from build123d import *

# Parameters (mm, degrees)
F0_R        = 63.5
F0_R_2      = 31.75
F1_DEPTH    = 25.4
F2_R        = 5.08
F3_R        = 5.08
F6_W        = 9.770580698
F6_H        = 10.6324088763
F6_W_2      = 13.55634837
F6_H_2      = 14.134524271
F7_DEPTH    = 25.4
F8_T1_DEPTH = 127.3817691468
F9_T1_DEPTH = 110.742504806


# Not quite as in the source:
# - a fillet or chamfer that OpenCascade refuses, or shapes differently, is made with other operations: its cross-section is extruded or revolved along the edge and cut away or added
# - the program builds the solid bodies; features that only make, move or delete a surface that nothing else refers to are left out


with BuildPart() as f1:
    # F0 (on Front) → F1 (new body)
    with BuildSketch(Plane.XZ):
        Circle(F0_R)
        Circle(F0_R_2, mode=Mode.SUBTRACT)
    extrude(amount=F1_DEPTH)

    # F2
    f2_edges = [f1.edges().sort_by_distance(p)[0] for p in [
        (-63.5, -25.4, 0),
    ]]
    fillet(f2_edges, radius=F2_R)

    # F3
    f3_edges = [f1.edges().sort_by_distance(p)[0] for p in [
        (-63.5, 0, 0),
    ]]
    fillet(f3_edges, radius=F3_R)

    # F6 (on face) → F7 (join)
    with BuildSketch(Plane.XZ.offset(25.4)):
        with Locations((34.2497480866, -27.0734353661)):
            Rectangle(F6_W, F6_H)
        with Locations((-26.7572421814, 31.0905136006)):
            Rectangle(F6_W_2, F6_H_2)
    extrude(amount=F7_DEPTH)

    # F8: fillet of radius 25.4 on 1 edges, made by hand

    # F8_s2 → F8_t1 (cut)
    with BuildSketch(Plane.YZ.offset(-90.4481267548)):
        with BuildLine():
            ThreePointArc((-28.0349158446, 38.1577757361), (-41.4329925067, 34.3367363635), (-50.8, 24.0232514651))
            Line((-50.8, 24.0232514651), (-50.8, 38.1577757361))
            Line((-50.8, 38.1577757361), (-28.0349158446, 38.1577757361))
        make_face()
    extrude(amount=F8_T1_DEPTH, mode=Mode.SUBTRACT)

    # F9: fillet of radius 25.4 on 1 edges, made by hand

    # F9_s2 → F9_t1 (cut)
    with BuildSketch(Plane.XY.offset(-82.4446877691)):
        with BuildLine():
            ThreePointArc((39.1350384356, -30.777980814), (36.5620755875, -41.9173872105), (29.3644577376, -50.8))
            Line((29.3644577376, -50.8), (39.1350384356, -50.8))
            Line((39.1350384356, -50.8), (39.1350384356, -30.777980814))
        make_face()
    extrude(amount=F9_T1_DEPTH, mode=Mode.SUBTRACT)


solid = f1.part
Check sheet for the modelled part. Datum: model origin and axes. Units: mm. A direction names the side the tool comes from. Give positions to 0.01 mm unless a question says otherwise; leave off trailing zeros. Order: outer loops, then holes, each group sorted by start corner. A loop starts at its lowest first (then second) coordinate and runs counter-clockwise, first axis right, second up. Notation, with made-up numbers: (86.25, -14) - (104.25, -14) arc R29 ccw to (104.25, 12) - close; hole circle Ø9 at (71, 83.25). An arc over 180 degrees is marked (long way). Answer as CSV lines item,"result".
1. Go/stop test with flat-tipped pins: P1, Ø3, axis at y = -40.5, z = 35.5, coming from the +X side; P2, Ø12, axis at x = 40, y = -11, coming from the -Z side; P3, Ø2, axis at y = -8.5, z = 34, coming from the +X side; P4, Ø12, axis at x = -2, z = -24, coming from the +Y side. Record where each tip stops, or that it passes through.
Result sheet:
P1,"x = -19.98"
P2,"z = -53.63"
P3,"x = 54.25"
P4,"through"
2. Tool access check on faces 4 (the face through (29.364, -38, -27)), 5 (the face through (33, -35, -32.39)), 6 (the face through (-19.979, -35, 29)), 7 (the face through (33, -35, -21.757)). Record the directions out of +Z, -Z, +X, -X, +Y, -Y that give a thin tool (end or side, any length) a straight path to the whole face; none if there is none.
Result sheet:
face 4,"+Z, -Z, -X, -Y"
face 5,"-Z, +X, -X, -Y"
face 6,"+Z, -Z, +X, -Y"
face 7,"+Z, +X, -X, -Y"
3. Scan lines: probe 1 along Z at (x, y) = (0, -10); probe 2 along Y at (x, z) = (1.5, 36); probe 3 along X at (y, z) = (-12.5, -1). Record each from-to range of solid material in increasing order. Write a range as from..to.
Result sheet:
probe 1,"-63.5..-31.75, 31.75..63.5"
probe 2,"-25.4..0"
probe 3,"-63.49..-31.73, 31.73..63.49"
4. Section check D-D (y = -14.5). Record the boundary of the cut face in (x, z).
Result sheet:
outline,"circle Ø127 at (0, 0); hole circle Ø63.5 at (0, 0)"
5. Section check C-C (y = -42). Record the boundary of the cut face in (x, z), then the cut area to 3 significant figures.
Result sheet:
outline,"(-33.54, 24.02) - (-19.98, 24.02) - (-19.98, 33.97) - (-33.54, 33.97) - close; (29.36, -32.39) - (36.52, -32.39) - (36.52, -21.76) - (29.36, -21.76) - close"
area,"211 mm²"
6. Mould release check, pull along Z, two halves, no side actions. Record for faces 1 (the face through (36.632, -41.772, -27.148)), 2 (the face through (-27, -38, 24.023)), 3 (the face through (-6.883, -12.522, -30.995)): released by +Z, released by -Z, zero draft, split by the parting line, or undercut.
Result sheet:
face 1,"zero draft"
face 2,"released by -Z"
face 3,"undercut"
7. Section check A-A (z = 0). Record the boundary of the cut face in (x, y), then the cut area to 3 significant figures.
Result sheet:
outline,"(-63.5, -20.32) arc R5.08 ccw to (-58.42, -25.4) - (-31.75, -25.4) - (-31.75, 0) - (-58.42, 0) arc R5.08 ccw to (-63.5, -5.08) - close; (31.75, -25.4) - (58.42, -25.4) arc R5.08 ccw to (63.5, -20.32) - (63.5, -5.08) arc R5.08 ccw to (58.42, 0) - (31.75, 0) - close"
area,"1,590 mm²"
8. Section check B-B (x = 0). Record the boundary of the cut face in (y, z), then the cut area to 3 significant figures.
Result sheet:
outline,"(-25.4, -58.42) arc R5.08 ccw to (-20.32, -63.5) - (-5.08, -63.5) arc R5.08 ccw to (0, -58.42) - (0, -31.75) - (-25.4, -31.75) - close; (-25.4, 31.75) - (0, 31.75) - (0, 58.42) arc R5.08 ccw to (-5.08, 63.5) - (-20.32, 63.5) arc R5.08 ccw to (-25.4, 58.42) - close"
area,"1,590 mm²"
